Check sheet for the drawn part. Datum: minimum x, y, z corner. Units: mm. Round coordinates to 2 decimals unless told otherwise and drop trailing zeros. Order: outer loops, then holes, each group sorted by start corner. A loop starts at its lowest first (then second) coordinate and runs counter-clockwise, first axis right, second up. Notation, with made-up numbers: (25.25, 18.25) -> (44.25, 18.25) arc R21 ccw to (44.25, 45.25) -> close; hole circle Ø3 at (56.5, 74). An arc over 180 degrees is marked (long way). Use CSV: the item, a comma, the result in double quotes.
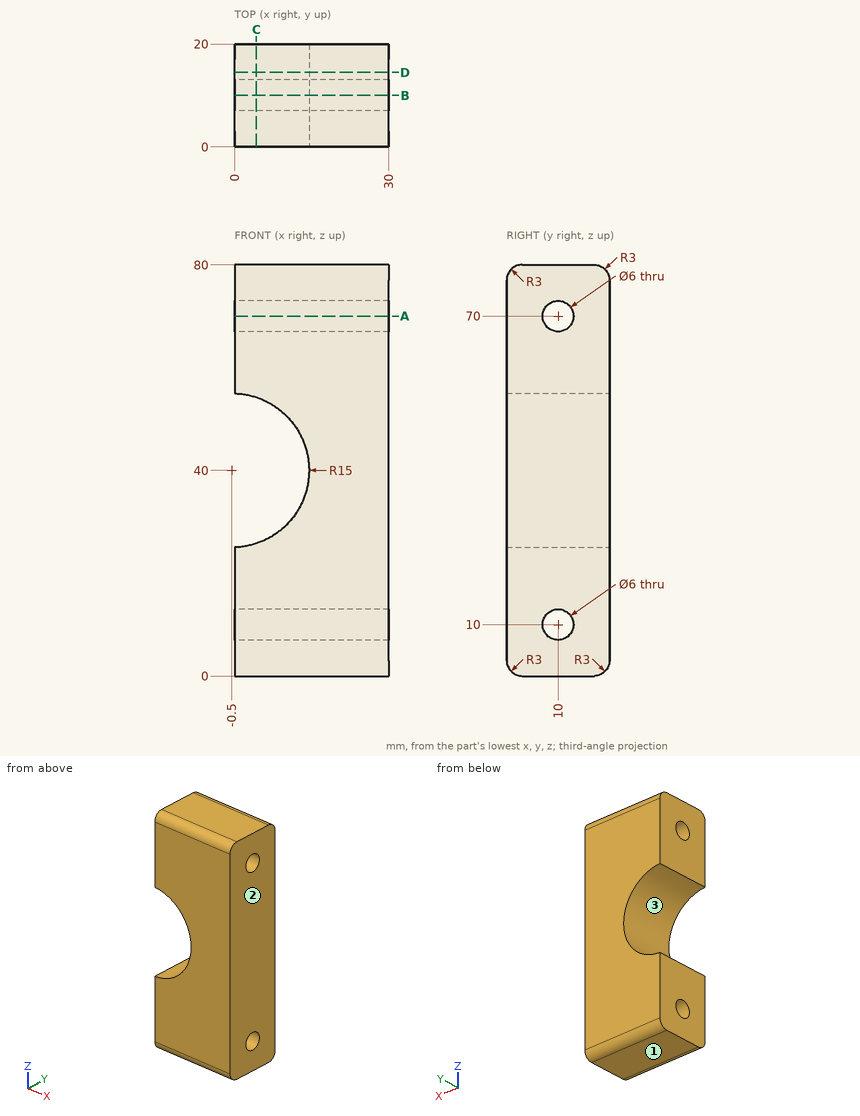
Q1. Sectioned sample at C-C, the plane x = 4.25. Enter the section's corners in (y, z).
Result sheet:
outline,"(0, 3) arc R3 ccw to (3, 0) -> (17, 0) arc R3 ccw to (20, 3) -> (20, 25.77) -> (0, 25.77) -> close; (0, 54.23) -> (20, 54.23) -> (20, 77) arc R3 ccw to (17, 80) -> (3, 80) arc R3 ccw to (0, 77) -> close; hole circle Ø6 at (10, 10); hole circle Ø6 at (10, 70)"
Q2. Sectioned sample at B-B, the plane y = 10. Enter the section's corners in (x, z).
Result sheet:
outline,"(0, 0) -> (30, 0) -> (30, 7) -> (0, 7) -> close; (0, 13) -> (30, 13) -> (30, 67) -> (0, 67) -> (0, 54.99) arc R15 cw to (0, 25.01) -> close; (0, 73) -> (30, 73) -> (30, 80) -> (0, 80) -> close"
Q3. Go/stop test with a flat-tipped pin: pin 1 (5 mm diameter, centred on x = 6, y = 17.5, fed in from -Z). Record where the tip stops, or that it passes through.
Result sheet:
pin 1,"stops at z = 0"
Q4. Sectioned sample at D-D, the plane y = 14.5. Enter the section's corners in (x, z), then the cut area to 3 significant figures.
Result sheet:
outline,"(0, 0) -> (30, 0) -> (30, 80) -> (0, 80) -> (0, 54.99) arc R15 cw to (0, 25.01) -> close"
area,"2,060 mm^2"
Q5. Mould release check, pull along Z, two halves, no side actions. Record for the marked faces 1, 2 and 3: pulls with the +Z half, pulls with the -Z half, needs draft (parallel to the pull), parting line crosses it, or undercut.
Result sheet:
face 1,"pulls with the -Z half"
face 2,"needs draft"
face 3,"undercut"
Q6. Scan lines: L1, parallel to Z at x = 16, y = 10; L2, parallel to Y at x = 8, z = 70; L3, parallel to Z at x = 23, y = 8.25. Record each from-to range of solid material in increasing order.
Result sheet:
L1,"z = 0 to 7, 13 to 67, 73 to 80"
L2,"y = 0 to 7, 13 to 20"
L3,"z = 0 to 7.56, 12.44 to 67.56, 72.44 to 80"
Q7. Sectioned sample at A-A, the plane z = 70. Enter the section's corners in (x, y).
Result sheet:
outline,"(0, 0) -> (30, 0) -> (30, 7) -> (0, 7) -> close; (0, 13) -> (30, 13) -> (30, 20) -> (0, 20) -> close"
